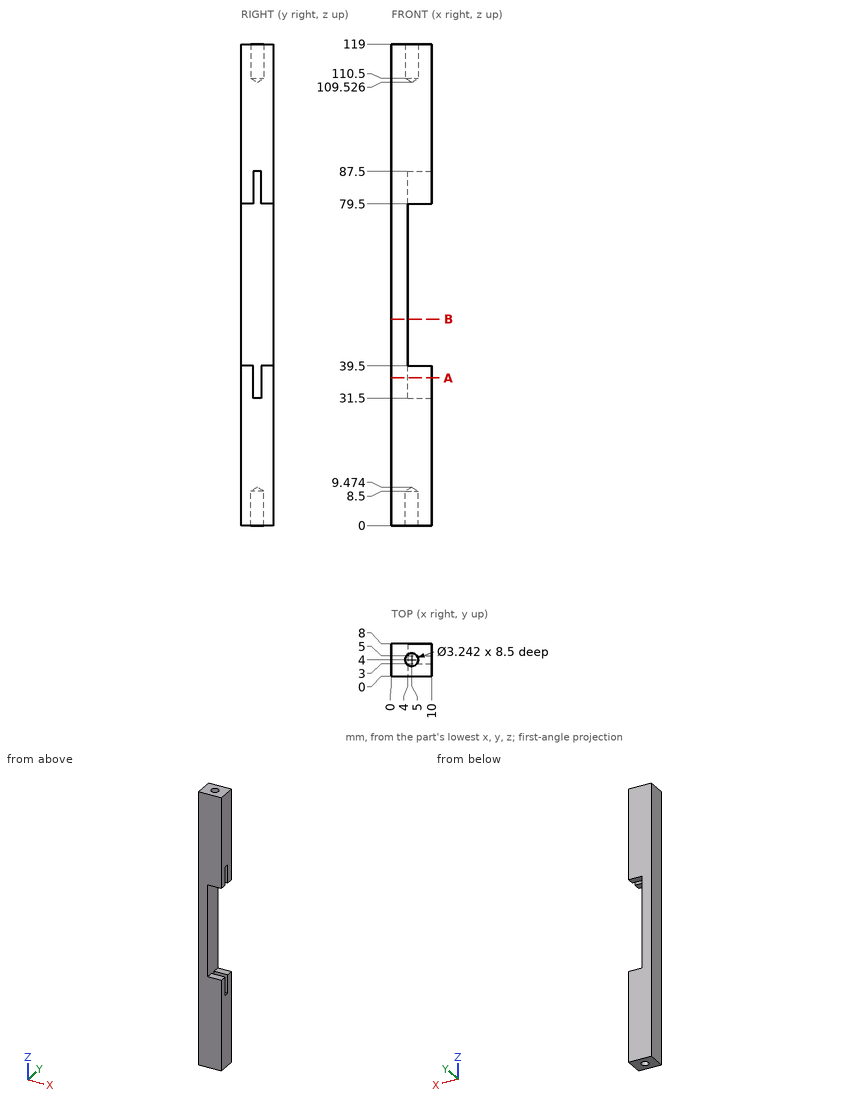
Here's the drawing with two shaded views (mm, measured from the low corner). I have some questions. Round coordinates to 2 decimals unless told otherwise and drop trailing zeros. Write each loop counter-clockwise with the first axis right and the second up, starting at its lowest first coordinate (ties: lowest second). Pieces come first, ordered by that corner, then holes.
(1) Suppose I cut it at B-B on z = 51. Write out the boundary of the cut face in (x, y), and give its area (3 significant figures).
Findings below:
outline: (0, 0) - (4, 0) - (4, 8) - (0, 8) - close
area: 32.0 mm2
(2) Suppose I cut it at A-A on z = 36.5. Write out the boundary of the cut face in (x, y), and give its area (3 significant figures).
Findings below:
outline: (0, 0) - (10, 0) - (10, 3) - (4, 3) - (4, 5) - (10, 5) - (10, 8) - (0, 8) - close
area: 68.0 mm2
(3) For pin 1 (3 mm diameter, centred on y = 3.5, z = 59, fed in from -X); pin 2 (1.9 mm diameter, centred on x = 5, y = 4, fed in from -Z), each with a flat end and sliding along its axis, tell me the tip position at first contact or that it passes through.
Findings below:
pin 1: stops at x = 0
pin 2: stops at z = 8.9
(4) If I drill on probe 1 along X at (y, z) = (4, 3); probe 2 along Z at (x, y) = (9.5, 1.75); probe 3 along Z at (x, y) = (8, 3.5), over which ranges is the centre line in solid material (lowest first)?
Findings below:
probe 1: x = 0 to 3.38, 6.62 to 10
probe 2: z = 0 to 39.5, 79.5 to 119
probe 3: z = 0 to 31.5, 87.5 to 119
